from build123d import *

# Parameters (mm, degrees)
SKETCH1_W           = 25
SKETCH1_H           = 88
BOSS_EXTRUDE1_DEPTH = 3
SKETCH2_R           = 1.5
CUT_EXTRUDE1_DEPTH  = 3
SKETCH3_W           = 3.2
SKETCH3_H           = 80
CUT_EXTRUDE2_DEPTH  = 10


with BuildPart() as part:
    # Sketch1 → Boss-Extrude1 (new body)
    with BuildSketch(Plane.XY):
        with Locations((12.5, 44)):
            Rectangle(SKETCH1_W, SKETCH1_H)
    extrude(amount=BOSS_EXTRUDE1_DEPTH)

    # Sketch2 → Cut-Extrude1 (cut)
    with BuildSketch(Plane.XY.offset(3)):
        with Locations((19, 82)):
            Circle(SKETCH2_R)
        with Locations((6, 82)):
            Circle(SKETCH2_R)
    extrude(amount=-CUT_EXTRUDE1_DEPTH, mode=Mode.SUBTRACT)

    # Sketch3 → Cut-Extrude2 (cut)
    with BuildSketch(Plane.XY.offset(3)):
        with Locations((12.5, 40)):
            Rectangle(SKETCH3_W, SKETCH3_H)
    extrude(amount=-CUT_EXTRUDE2_DEPTH, mode=Mode.SUBTRACT)


solid = part.part
Can you work these out from the model? Positions are in its coordinate system, mm. A direction names the side the tool comes from. Give positions to 0.01 mm unless a question says otherwise; leave off trailing zeros. Order: outer loops, then holes, each group sorted by start corner. A loop starts at its lowest first (then second) coordinate and runs counter-clockwise, first axis right, second up. Notation, with made-up numbers: M -40,42.5 L -8,42.5 A31 cw -8,79.5 Z; hole C 67,-26.75 d5. An arc over 180 degrees is marked long. Use one line per item in the form item = value. Start each with the question number.
Item 1: If we section it at C-C (y = 66): Write out the boundary of the cut face in (x, z), then the cut area to 3 significant figures.
Item 2: If we section it at A-A (z = 2.2): Write out the boundary of the cut face in (x, y).
Item 3: We'd pull the mould along Y, two halves only. Please class faces 1 (the flat face through (0, 43, 1)), 2 (the flat face through (12, 88, 1)), 3 (the flat face through (12, 80, 2)), 4 (the cylindrical face through (5.805, 83.487, 1.521)): +Y half, -Y half, draft (parallel to the pull), parting line (faces both ways), or undercut.
Item 4: If we section it at B-B (x = 19): Write out the boundary of the cut face in (y, z), then the cut area to 3 significant figures.
Item 5: For faces 5 (the flat face through (25, 43, 1)), 6 (the flat face through (14.1, 39, 2)), which set-ups out of +Z, -Z, +X, -X, +Y, -Y let a thin tool reach every point of the face, with its end or its side?
Item 6: If I drill on line 1 along X through (y, z) = (82, 2.2); line 2 along X through (y, z) = (51.5, 2.35); line 3 along Y through (x, z) = (6, 0.7), over which ranges is the centre line in solid material (lowest first)?
Item 7: If we section it at D-D (y = 82): Write out the boundary of the cut face in (x, z), then the cut area to 3 significant figures.
Outcome:
q1.outline = M 0,0 L 10.9,0 L 10.9,3 L 0,3 Z; M 14.1,0 L 25,0 L 25,3 L 14.1,3 Z
q1.area = 65.4 mm2
q2.outline = M 0,0 L 10.9,0 L 10.9,80 L 14.1,80 L 14.1,0 L 25,0 L 25,88 L 0,88 Z; hole C 6,82 d3; hole C 19,82 d3
q3.face_1 = draft
q3.face_2 = +Y half
q3.face_3 = -Y half
q3.face_4 = undercut
q4.outline = M 0,0 L 80.5,0 L 80.5,3 L 0,3 Z; M 83.5,0 L 88,0 L 88,3 L 83.5,3 Z
q4.area = 255 mm2
q5.face_5 = +Z, -Z, +X, +Y, -Y
q5.face_6 = +Z, -Z, -Y
q6.line_1 = 0 to 4.5, 7.5 to 17.5, 20.5 to 25
q6.line_2 = 0 to 10.9, 14.1 to 25
q6.line_3 = 0 to 80.5, 83.5 to 88
q7.outline = M 0,0 L 4.5,0 L 4.5,3 L 0,3 Z; M 7.5,0 L 17.5,0 L 17.5,3 L 7.5,3 Z; M 20.5,0 L 25,0 L 25,3 L 20.5,3 Z
q7.area = 57.0 mm2
